Could you check a few things on this model? Use its own coordinates, in mm. Face numbers are marked on the shaded views. A direction names the side the tool comes from. Give positions to 0.01 mm unless a question says otherwise; leave off trailing zeros. Write each loop counter-clockwise with the first axis right and the second up, starting at its lowest first coordinate (ties: lowest second). Pieces come first, ordered by that corner, then holes. Notation, with made-up numbers: (-32, -4) -> (-5, -4) arc R11 ccw to (-5, 12) -> close; hole circle Ø9 at (85.5, 21). An arc over 180 degrees is marked (long way). One line per question, with ' | ' between items.
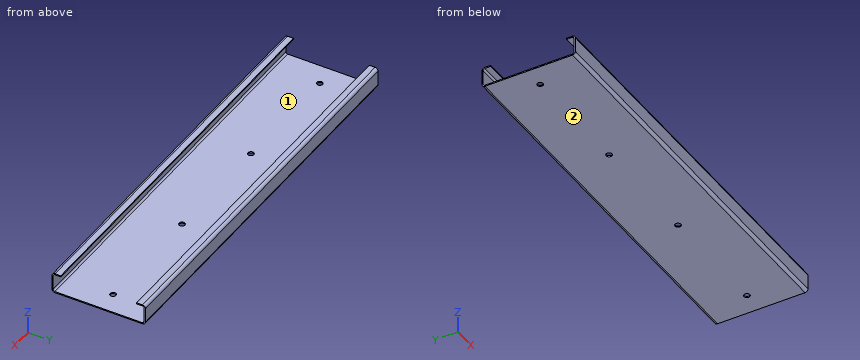
from build123d import *

# Parameters (mm, degrees)
SKETCH1_W                      = 675
SKETCH1_H                      = 160
BASE_FLANGE1_DEPTH             = 2
EDGE_FLANGE1_STRIP_W           = 14
EDGE_FLANGE1_STRIP_H           = 2
EDGE_FLANGE1_STRIP_CUT_DEPTH   = 675
EDGE_FLANGE1_STRIP_2_W         = 14
EDGE_FLANGE1_STRIP_2_H         = 2
EDGE_FLANGE1_STRIP_CUT_2_DEPTH = 675
EDGE_FLANGE1_DEPTH             = 675
EDGE_FLANGE1_BEND_DEPTH        = 675
EDGE_FLANGE2_STRIP_W           = 14
EDGE_FLANGE2_STRIP_H           = 2
EDGE_FLANGE2_STRIP_CUT_DEPTH   = 675
EDGE_FLANGE2_STRIP_2_W         = 14
EDGE_FLANGE2_STRIP_2_H         = 2
EDGE_FLANGE2_STRIP_CUT_2_DEPTH = 675
EDGE_FLANGE2_DEPTH             = 675
EDGE_FLANGE2_BEND_DEPTH        = 675
SKETCH18_R                     = 5
CUT_EXTRUDE1_DEPTH             = 10
LPATTERN1_COUNT                = 4
LPATTERN1_PITCH                = 200


# Sheet-metal steps are written as plain solids
with BuildPart() as part:
    # Sketch1 → Base-Flange1 (new body)
    with BuildSketch(Plane.XY):
        Rectangle(SKETCH1_W, SKETCH1_H)
    extrude(amount=-BASE_FLANGE1_DEPTH)

    # Edge-Flange1 strip (across the edge) → Edge-Flange1 strip cut (cut)
    with BuildSketch(Plane(origin=(337.5, 80, 0), x_dir=(0, -1, 0), z_dir=(-1, 0, 0))):
        with Locations((-2, -1)):
            Rectangle(EDGE_FLANGE1_STRIP_W, EDGE_FLANGE1_STRIP_H)
    extrude(amount=EDGE_FLANGE1_STRIP_CUT_DEPTH, mode=Mode.SUBTRACT)

    # Edge-Flange1 strip 2 (across the edge) → Edge-Flange1 strip cut 2 (cut)
    with BuildSketch(Plane(origin=(-337.5, -80, 0), x_dir=(0, 1, 0), z_dir=(1, 0, 0))):
        with Locations((-2, -1)):
            Rectangle(EDGE_FLANGE1_STRIP_2_W, EDGE_FLANGE1_STRIP_2_H)
    extrude(amount=EDGE_FLANGE1_STRIP_CUT_2_DEPTH, mode=Mode.SUBTRACT)

    # Edge-Flange1 section (across the edge) → Edge-Flange1 (add)
    with BuildSketch(Plane(origin=(337.5, 80, 0), x_dir=(0, -1, 0), z_dir=(-1, 0, 0))):
        with BuildLine():
            Line((0, 3), (0, 33))
            Line((0, 33), (2, 33))
            Line((2, 33), (2, 3))
            ThreePointArc((2, 3), (2.878679656, 0.878679656), (5, 0))
            Line((5, 0), (5, -2))
            ThreePointArc((5, -2), (1.464466094, -0.535533906), (0, 3))
        make_face()
    extrude(amount=EDGE_FLANGE1_DEPTH)

    # Edge-Flange1 section 2 (across the edge) → Edge-Flange1 bend (add)
    with BuildSketch(Plane(origin=(-337.5, -80, 0), x_dir=(0, 1, 0), z_dir=(1, 0, 0))):
        with BuildLine():
            Line((0, 3), (0, 33))
            Line((0, 33), (2, 33))
            Line((2, 33), (2, 3))
            ThreePointArc((2, 3), (2.878679656, 0.878679656), (5, 0))
            Line((5, 0), (5, -2))
            ThreePointArc((5, -2), (1.464466094, -0.535533906), (0, 3))
        make_face()
    extrude(amount=EDGE_FLANGE1_BEND_DEPTH)

    # Edge-Flange2 strip (across the edge) → Edge-Flange2 strip cut (cut)
    with BuildSketch(Plane(origin=(-337.5, -78, 33), x_dir=(0, 0, -1), z_dir=(1, 0, 0))):
        with Locations((-2, -1)):
            Rectangle(EDGE_FLANGE2_STRIP_W, EDGE_FLANGE2_STRIP_H)
    extrude(amount=EDGE_FLANGE2_STRIP_CUT_DEPTH, mode=Mode.SUBTRACT)

    # Edge-Flange2 strip 2 (across the edge) → Edge-Flange2 strip cut 2 (cut)
    with BuildSketch(Plane(origin=(337.5, 78, 33), x_dir=(0, 0, -1), z_dir=(-1, 0, 0))):
        with Locations((-2, -1)):
            Rectangle(EDGE_FLANGE2_STRIP_2_W, EDGE_FLANGE2_STRIP_2_H)
    extrude(amount=EDGE_FLANGE2_STRIP_CUT_2_DEPTH, mode=Mode.SUBTRACT)

    # Edge-Flange2 section (across the edge) → Edge-Flange2 (add)
    with BuildSketch(Plane(origin=(-337.5, -78, 33), x_dir=(0, 0, -1), z_dir=(1, 0, 0))):
        with BuildLine():
            Line((0, 3), (0, 13))
            Line((0, 13), (2, 13))
            Line((2, 13), (2, 3))
            ThreePointArc((2, 3), (2.878679656, 0.878679656), (5, 0))
            Line((5, 0), (5, -2))
            ThreePointArc((5, -2), (1.464466094, -0.535533906), (0, 3))
        make_face()
    extrude(amount=EDGE_FLANGE2_DEPTH)

    # Edge-Flange2 section 2 (across the edge) → Edge-Flange2 bend (add)
    with BuildSketch(Plane(origin=(337.5, 78, 33), x_dir=(0, 0, -1), z_dir=(-1, 0, 0))):
        with BuildLine():
            Line((0, 3), (0, 13))
            Line((0, 13), (2, 13))
            Line((2, 13), (2, 3))
            ThreePointArc((2, 3), (2.878679656, 0.878679656), (5, 0))
            Line((5, 0), (5, -2))
            ThreePointArc((5, -2), (1.464466094, -0.535533906), (0, 3))
        make_face()
    extrude(amount=EDGE_FLANGE2_BEND_DEPTH)

    # Sketch18 → Cut-Extrude1 (cut)
    with BuildSketch(Plane(origin=(0, 0, -2), x_dir=(-1, 0, 0), z_dir=(0, 0, -1))):
        with Locations((-300, 2.49)):
            Circle(SKETCH18_R)
    cut_extrude1 = extrude(amount=-CUT_EXTRUDE1_DEPTH, mode=Mode.SUBTRACT)

    # LPattern1: Cut-Extrude1 ×4
    with Locations(*[(-i * LPATTERN1_PITCH, 0, 0) for i in range(1, LPATTERN1_COUNT)]):
        add(cut_extrude1, mode=Mode.SUBTRACT)


solid = part.part
Q1. Imagine slicing it at B-B on x = -184.5. Please give me the cut outline in (y, z), and give its area (3 significant figures).
Answer below:
outline: (-80, 3) arc R5 ccw to (-75, -2) -> (75, -2) arc R5 ccw to (80, 3) -> (80, 28) arc R5 ccw to (75, 33) -> (65, 33) -> (65, 31) -> (75, 31) arc R3 cw to (78, 28) -> (78, 3) arc R3 cw to (75, 0) -> (-75, 0) arc R3 cw to (-78, 3) -> (-78, 28) arc R3 cw to (-75, 31) -> (-65, 31) -> (-65, 33) -> (-75, 33) arc R5 ccw to (-80, 28) -> close | area: 490 mm^2
Q2. On a 3-axis mill with a long thin cutter (end or side, diameter ignored), from which of +Z, -Z, +X, -X, +Y, -Y can I reach the whole of each face in a straight line? I mean the marked faces 1 and 2. Say none if no direction works.
Answer below:
face 1: +X, -X | face 2: -Z, +X, -X, +Y, -Y
Q3. Will these pins go through, and if not, where does the flat tip stop? pin 1 (10 mm diameter, centred on y = -17.5, z = 6, fed in from -X); pin 2 (4 mm diameter, centred on x = -245.5, y = 51, fed in from +Z); pin 3 (1.6 mm diameter, centred on x = -125, z = 31.5, fed in from +Y); pin 4 (0.6 mm diameter, centred on x = 6.5, z = 32.5, fed in from -Y).
Answer below:
pin 1: passes through | pin 2: stops at z = 0 | pin 3: stops at y = 79.21 | pin 4: stops at y = -77.71
Q4. Imagine slicing it at C-C on y = -46. Please give me the cut outline in (x, z), and give its area (3 significant figures).
Answer below:
outline: (-337.5, -2) -> (337.5, -2) -> (337.5, 0) -> (-337.5, 0) -> close | area: 1,350 mm^2
Q5. Imagine slicing it at A-A on z = 14.5. Please give me the cut outline in (x, y).
Answer below:
outline: (-337.5, -80) -> (337.5, -80) -> (337.5, -78) -> (-337.5, -78) -> close; (-337.5, 78) -> (337.5, 78) -> (337.5, 80) -> (-337.5, 80) -> close
Q6. If I drill on line 1 along X through (y, z) = (2, -1); line 2 along Y through (x, z) = (298.5, 18); line 3 along Y through (x, z) = (-300, -0.95), over which ranges is the centre line in solid material (lowest first)?
Answer below:
line 1: x = -337.5 to -304.98, -295.02 to -104.98, -95.02 to 95.02, 104.98 to 295.02, 304.98 to 337.5 | line 2: y = -80 to -78, 78 to 80 | line 3: y = -78.07 to -2.51, 7.49 to 78.07
